```python
from build123d import *

# Parameters (mm, degrees)
SKETCH_396_R           = 7.6
EXTRUDE_924_DEPTH      = 15
CUT_EXTRUDE_1360_DEPTH = 10
SKETCH_1871_R          = 7.6
EXTRUDE_2829_DEPTH     = 10
SKETCH_2885_R          = 7.6
CUT_EXTRUDE_3705_DEPTH = 15.5
SKETCH_7625_R          = 9.15
SKETCH_7625_R_2        = 7.65
EXTRUDE_7744_DEPTH     = 0.5


with BuildPart() as part:
    # Sketch 396 → Extrude 924 (new body)
    with BuildSketch(Plane.XY):
        with BuildLine():
            Line((33.023854242, 2.889212872), (32.0215632, 14.3454519))
            Line((32.0215632, 14.3454519), (35.508244643, 14.650497))
            Line((35.508244643, 14.650497), (33.329351075, 39.555364452))
            Line((33.329351075, 39.555364452), (56.241829131, 41.559946535))
            Line((56.241829131, 41.559946535), (58.4207227, 16.655079083))
            Line((58.4207227, 16.655079083), (61.907404143, 16.960124183))
            Line((61.907404143, 16.960124183), (62.909695184, 5.503885155))
            ThreePointArc((62.909695184, 5.503885155), (46.55906382, -42.663521611), (0, -63.15))
            ThreePointArc((0, -63.15), (-15, -48.15), (0, -33.15))
            ThreePointArc((0, -33.15), (24.440743715, -22.395815382), (33.023854242, 2.889212872))
        make_face()
        with Locations((0, -48.15)):
            Circle(SKETCH_396_R, mode=Mode.SUBTRACT)
    extrude(amount=EXTRUDE_924_DEPTH)

    # Sketch 979 → Cut-Extrude 1360 (cut)
    with BuildSketch(Plane(origin=(62.909695184, 5.503885155, 0), x_dir=(0, 0, -1), z_dir=(0.9961946980917458, 0.08715574274765542, 0))):
        with BuildLine():
            ThreePointArc((-6.5, 30), (-6.792893219, 30.707106781), (-7.5, 31))
            Line((-7.5, 31), (-7.5, 29))
            ThreePointArc((-7.5, 29), (-6.792893219, 29.292893219), (-6.5, 30))
        make_face()
        with BuildLine():
            Line((-7.5, 29), (-7.5, 31))
            ThreePointArc((-7.5, 31), (-8.5, 30), (-7.5, 29))
        make_face()
        with BuildLine():
            ThreePointArc((-6.5, 18), (-6.792893219, 18.707106781), (-7.5, 19))
            Line((-7.5, 19), (-7.5, 17))
            ThreePointArc((-7.5, 17), (-6.792893219, 17.292893219), (-6.5, 18))
        make_face()
        with BuildLine():
            Line((-7.5, 17), (-7.5, 19))
            ThreePointArc((-7.5, 19), (-8.5, 18), (-7.5, 17))
        make_face()
    cut_extrude_1360 = extrude(amount=-CUT_EXTRUDE_1360_DEPTH, mode=Mode.SUBTRACT)

    # Mirror 1436: Cut-Extrude 1360 across plane
    add(cut_extrude_1360.mirror(Plane(origin=(47.966774713, 4.196549013, 0), x_dir=(0, 0, 1), z_dir=(0.9961946980917455, 0.0871557427476578, 0))), mode=Mode.SUBTRACT)

    # Sketch 1871 → Extrude 2829 (add)
    with BuildSketch(Plane.XY.offset(15)):
        with BuildLine():
            ThreePointArc((0, -63.15), (22.275075929, -59.090976404), (41.686650392, -47.43570047))
            ThreePointArc((41.686650392, -47.43570047), (43.052220482, -26.26649599), (21.883016002, -24.9009259))
            ThreePointArc((21.883016002, -24.9009259), (11.693092115, -31.019253647), (0, -33.15))
            ThreePointArc((0, -33.15), (-15, -48.15), (0, -63.15))
        make_face()
        with Locations((0, -48.15)):
            Circle(SKETCH_1871_R, mode=Mode.SUBTRACT)
    extrude(amount=EXTRUDE_2829_DEPTH)

    # Sketch 2885 → Cut-Extrude 3705 (cut)
    with BuildSketch(Plane(origin=(0, 0, 0), x_dir=(-1, 0, 0), z_dir=(0, 0, -1))):
        with BuildLine():
            ThreePointArc((0, -63.15), (15, -48.15), (0, -33.15))
            ThreePointArc((0, -33.15), (-10.671339307, -31.385426831), (-20.206608689, -26.279563643))
            ThreePointArc((-20.206608689, -26.279563643), (-17.458666259, -47.314030755), (-38.493133336, -50.061973453))
            ThreePointArc((-38.493133336, -50.061973453), (-20.328660512, -59.788527844), (0, -63.15))
        make_face()
        with Locations((0, -48.15)):
            Circle(SKETCH_2885_R, mode=Mode.SUBTRACT)
    extrude(amount=-CUT_EXTRUDE_3705_DEPTH, mode=Mode.SUBTRACT)

    # Sketch 7625 → Extrude 7744 (add)
    with BuildSketch(Plane.XY.offset(25)):
        with Locations((0, -48.15)):
            Circle(SKETCH_7625_R)
        with Locations((0, -48.15)):
            Circle(SKETCH_7625_R_2, mode=Mode.SUBTRACT)
    extrude(amount=EXTRUDE_7744_DEPTH)


solid = part.part
```
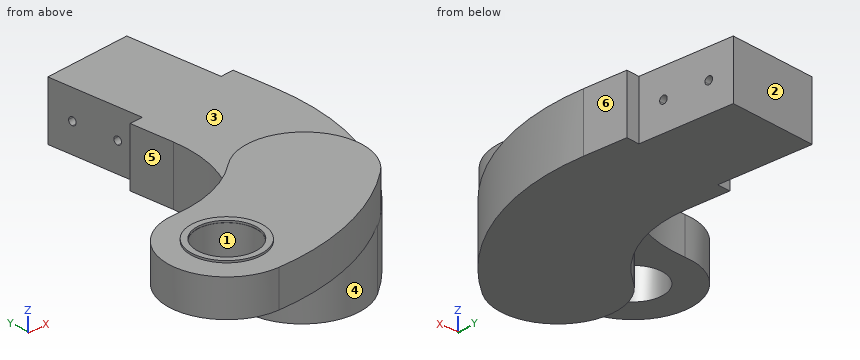
For this review, take the finished solid that the model builds, in its own axes (mm). Face numbers are marked on the shaded views. A direction names the side the tool comes from. Round coordinates to 2 decimals unless told otherwise and drop trailing zeros. Write each loop counter-clockwise with the first axis right and the second up, starting at its lowest first coordinate (ties: lowest second). Pieces come first, ordered by that corner, then holes.
1) For line 1 along Y through (x, z) = (0, 20.5); line 2 along Y through (x, z) = (0, 25.3); line 3 along Z through (x, y) = (29.5, -41.5), list the stretches that pass through material, from the lowest coordinate up.
Answer below:
line 1: y = -63.15 to -55.75, -40.55 to -33.15
line 2: y = -57.3 to -55.8, -40.5 to -39
line 3: z = 0 to 25
2) Mouldability with a two-part tool opening along Y and no side actions: class the marked faces 1, 2 and 3 as +Y half, -Y half, draft (parallel to the pull), parting line (faces both ways), or undercut.
Answer below:
face 1: undercut
face 2: +Y half
face 3: draft
3) Machinability: for the marked faces 4, 5 and 6, which of the approach directions +Z, -Z, +X, -X, +Y, -Y give a long, thin tool a straight path to every point of the face, cutting with its end or side? Answer none if there is none.
Answer below:
face 4: -Z
face 5: +Z, -Z, -X
face 6: +Z, -Z, +X, +Y
4) Take a section at D-D on x = 27.5. Give the boundary of the cut face in (y, z), then the cut area to 3 significant figures.
Answer below:
outline: (-56.85, 15.5) - (-53.06, 15.5) - (-53.06, 0) - (-18.51, 0) - (-18.51, 15) - (-21.79, 15) - (-21.79, 25) - (-56.85, 25) - close
area: 867 mm2
5) Insertion check: pin 1 Ø6 at (y, z) = (-5, 4.5) entering from -X; pin 2 Ø1 at (y, z) = (-49.5, 14.5) entering from +X; pin 3 Ø20 at (x, y) = (0, -48.15) entering from -Z; pin 4 Ø2 at (x, y) = (48.5, -6) entering from -Z. Each pin has a flat end and moves straight along its axis. Give the tip position at first contact, or say it passes through.
Answer below:
pin 1: stops at x = 32.17
pin 2: stops at x = 39.84
pin 3: stops at z = 15.5
pin 4: stops at z = 0
6) Take a section at B-B on x = 3. Give the boundary of the cut face in (y, z).
Answer below:
outline: (-63.08, 15.5) - (-55.13, 15.5) - (-55.13, 25) - (-55.19, 25) - (-55.19, 25.5) - (-56.79, 25.5) - (-56.79, 25) - (-63.08, 25) - close; (-41.17, 15.5) - (-33.01, 15.5) - (-33.01, 25) - (-39.51, 25) - (-39.51, 25.5) - (-41.11, 25.5) - (-41.11, 25) - (-41.17, 25) - close
7) Take a section at C-C on z = 20. Give the boundary of the cut face in (x, y).
Answer below:
outline: (0, -63.15) arc R63.15 ccw to (41.69, -47.44) arc R15 ccw to (21.88, -24.9) arc R33.15 cw to (0, -33.15) arc R15 ccw to start; hole circle Ø15.2 at (0, -48.15)
8) Take a section at A-A on z = 12.75. Give the boundary of the cut face in (x, y), then the cut area to 3 significant figures.
Answer below:
outline: (20.21, -26.28) arc R15 ccw to (38.49, -50.06) arc R63.15 ccw to (62.91, 5.5) - (61.91, 16.96) - (58.42, 16.66) - (56.24, 41.56) - (33.33, 39.56) - (35.51, 14.65) - (32.02, 14.35) - (33.02, 2.89) arc R33.15 cw to start
area: 2,720 mm2
